from build123d import *

# Parameters (mm, degrees)
F0_W      = 42
F0_H      = 27
F1_DEPTH  = 9
F2_W      = 32
F2_H      = 23
F3_DEPTH  = 7
F6_W      = 6
F6_H      = 7.5
F7_DEPTH  = 4
F5_W      = 6
F5_H      = 7.5
F10_DEPTH = 4
F12_DEPTH = 5
F14_R     = 2
F15_R     = 5


with BuildPart() as f1:
    # F0 (on Top) → F1 (new body)
    with BuildSketch(Plane.XY):
        Rectangle(F0_W, F0_H)
    extrude(amount=-F1_DEPTH)


with BuildPart() as f3:
    # F2 (on Top) → F3 (new body)
    with BuildSketch(Plane.XY):
        with Locations((5, 0)):
            Rectangle(F2_W, F2_H)
    extrude(amount=-F3_DEPTH)


with BuildPart() as f1_1:
    add(f1.part)

    # F4: cut F3
    add(f3.part, mode=Mode.SUBTRACT)


with BuildPart() as f7:
    # F6 (on Top) → F7 (new body)
    with BuildSketch(Plane.XY):
        with Locations((-14, -7.75)):
            Rectangle(F6_W, F6_H)
    extrude(amount=-F7_DEPTH)


with BuildPart() as f7b:
    # F5 (on Top) → F7, piece 2 (new body)
    with BuildSketch(Plane.XY):
        with Locations((-14, 7.75)):
            Rectangle(F5_W, F5_H)
    extrude(amount=-F7_DEPTH)


with BuildPart() as f1_2:
    add(f1_1.part)

    # F8: cut F7b, F7
    add(f7b.part, mode=Mode.SUBTRACT)
    add(f7.part, mode=Mode.SUBTRACT)

    # F9 (on face) → F10 (join)
    with BuildSketch(Plane(origin=(-21, 0, 0), x_dir=(0, -1, 0), z_dir=(-1, 0, 0))):
        Polygon((-13.5, 0), (13.5, 0), (33.5, 34.6410161514), (-33.5, 34.6410161514), align=None)
    extrude(amount=-F10_DEPTH)


with BuildPart() as f12:
    # F11 (on face) → F12 (new body)
    with BuildSketch(Plane(origin=(-21, 0, 0), x_dir=(0, -1, 0), z_dir=(-1, 0, 0))):
        Polygon((-7.5, 0), (7.5, 0), (27.5, 34.6410161514), (-27.5, 34.6410161514), align=None)
    extrude(amount=-F12_DEPTH)


with BuildPart() as f1_3:
    add(f1_2.part)

    # F13: cut F12
    add(f12.part, mode=Mode.SUBTRACT)

    # F14
    f14_edges = [f1_3.edges().sort_by_distance(p)[0] for p in [
        (-19, 33.5, 34.641016),
        (-19, 27.5, 34.641016),
        (-19, -27.5, 34.641016),
        (-19, -33.5, 34.641016),
        (-19, -7.5, 0),
        (-19, 7.5, 0),
        (-11, 0, 0),
        (-11, 7.75, -4),
        (-11, -7.75, -4),
    ]]
    fillet(f14_edges, radius=F14_R)

    # F15
    f15_edges = [f1_3.edges().sort_by_distance(p)[0] for p in [
        (-17, -12.5, 0),
        (-17, 12.5, 0),
        (21, 12.5, 0),
        (21, -12.5, 0),
    ]]
    fillet(f15_edges, radius=F15_R)


solid = f1_3.part
Source: CAD feature listing. Evaluate the final solid. Frame: model axes, mm. A direction names the side the tool comes from. Give positions to 0.01 mm unless a question says otherwise; leave off trailing zeros. Write each loop counter-clockwise with the first axis right and the second up, starting at its lowest first coordinate (ties: lowest second). Pieces come first, ordered by that corner, then holes. Notation, with made-up numbers: M 73.5,22 L 119.5,22 A28 ccw 119.5,61 Z; hole C -21,-12.5 d9. An arc over 180 degrees is marked long. Answer as a JSON object with one key per item and string values.
Q1. Access query for faces 1 (the face through (0, -13.5, -4)), 2 (the face through (2, 13, 0)), 3 (the face through (-19.028, -17.368, 17.092)), 4 (the face through (-15, 8, -4)). Directions: +Z, -Z, +X, -X, +Y, -Y. A direction counts if a zero-diameter tool reaches every point of the face in a straight line with its end or side. Return the directions, or none.
Geometry check:
{"face 1": "-Z, +X, -X, -Y", "face 2": "+Z, +X, +Y, -Y", "face 3": "+Z, +X, -X", "face 4": "+Z, +X"}
Q2. Cut plane A-A, the plane z = 30.5. Return the cut outline in (x, y), then the cut area to 3 significant figures.
Geometry check:
{"outline": "M -21,-31.11 L -17,-31.11 L -17,-25.11 L -21,-25.11 Z; M -21,25.11 L -17,25.11 L -17,31.11 L -21,31.11 Z", "area": "48.0 mm^2"}
Q3. Contact query for flat-ended pins moving along their axis: P1, Ø8.5, axis at y = 23, z = 9, coming from the +X side; P2, Ø1.2, axis at x = -15, y = -6, coming from the +Z side; P3, Ø5, axis at x = -14.5, z = -3, coming from the -Y side; P4, Ø8, axis at y = 13.5, z = 20.5, coming from the +X side. Output: stop coordinate, or through.
Geometry check:
{"P1": "stops at x = -17", "P2": "stops at z = -4", "P3": "stops at y = -13.5", "P4": "passes through"}
Q4. Ray query, line 1 along Y through (x, z) = (-7, -4); line 2 along X through (y, z) = (17.5, 13); line 3 along Z through (x, y) = (8, 7). Return the intervals inside material, ascending.
Geometry check:
{"line 1": "y = -13.5 to -11.5, 11.5 to 13.5", "line 2": "x = -21 to -17", "line 3": "z = -9 to -7"}
Q5. Cut plane B-B, the plane y = 5. Return the cut outline in (x, z).
Geometry check:
{"outline": "M -21,-9 L 21,-9 L 21,-7 L -11,-7 L -11,-6 A2 ccw -13,-4 L -17,-4 L -17,0 L -21,0 Z"}
Q6. Cut plane D-D, the plane z = -3. Return the cut outline in (x, y).
Geometry check:
{"outline": "M -21,-13.5 L 20.58,-13.5 L 20.58,-11.5 L -17,-11.5 L -17,-4 L -11,-4 L -11,4 L -17,4 L -17,11.5 L 20.58,11.5 L 20.58,13.5 L -21,13.5 Z"}
Q7. Cut plane C-C, the plane x = -10. Return the cut outline in (y, z), then the cut area to 3 significant figures.
Geometry check:
{"outline": "M -13.5,-9 L 13.5,-9 L 13.5,0 L 11.5,0 L 11.5,-7 L -11.5,-7 L -11.5,0 L -13.5,0 Z", "area": "82.0 mm^2"}
